Here's the drawing with two shaded views (mm, measured from the low corner). I have some questions. Coordinates: 2 decimals unless noted, no trailing zeros. Write each loop counter-clockwise with the first axis right and the second up, starting at its lowest first coordinate (ties: lowest second). Pieces come first, ordered by that corner, then holes. Notation, with made-up numbers: (27, 88.5) -> (66, 88.5) arc R17 ccw to (66, 105.5) -> close; hole circle Ø2 at (49.5, 72). An arc over 180 degrees is marked (long way). Put each result on its own line as item: value.
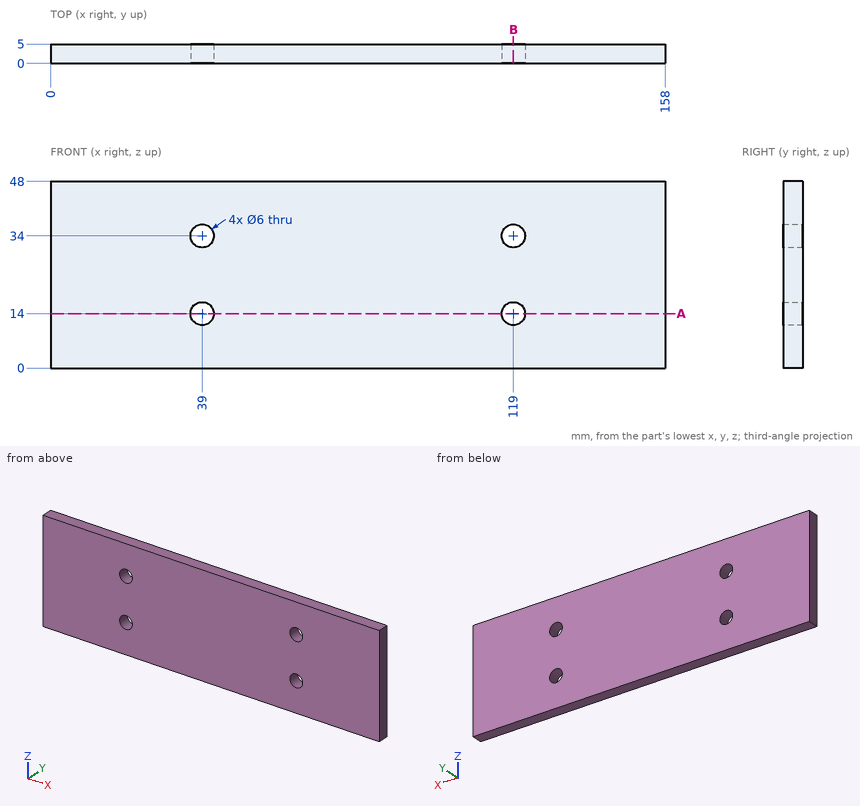
Item 1: Imagine slicing it at B-B on x = 119. Write out the boundary of the cut face in (y, z).
Output:
outline: (0, 0) -> (5, 0) -> (5, 11) -> (0, 11) -> close; (0, 17) -> (5, 17) -> (5, 31) -> (0, 31) -> close; (0, 37) -> (5, 37) -> (5, 48) -> (0, 48) -> close
Item 2: For P1, Ø5.5, axis at x = 39, z = 14, coming from the +Y side, with a flat end and sliding along its axis, tell me the tip position at first contact or that it passes through.
Output:
P1: passes through
Item 3: Please list where these lines run through material, in increasing order: line 1 along X through (y, z) = (1, 14); line 2 along X through (y, z) = (1.1, 35); line 3 along Z through (x, y) = (120, 4.6). Write a range as from..to.
Output:
line 1: x = 0..36, 42..116, 122..158
line 2: x = 0..36.17, 41.83..116.17, 121.83..158
line 3: z = 0..11.17, 16.83..31.17, 36.83..48
Item 4: Imagine slicing it at A-A on z = 14. Write out the boundary of the cut face in (x, y), then the cut area to 3 significant figures.
Output:
outline: (0, 0) -> (36, 0) -> (36, 5) -> (0, 5) -> close; (42, 0) -> (116, 0) -> (116, 5) -> (42, 5) -> close; (122, 0) -> (158, 0) -> (158, 5) -> (122, 5) -> close
area: 730 mm²
